```python
from build123d import *

# Parameters (mm, degrees)
SKETCH2_OUTSIDE_W   = 82.784
SKETCH2_OUTSIDE_H   = 82.784
SKETCH2_OUTSIDE_W_2 = 55
SKETCH2_OUTSIDE_H_2 = 76.69931098
CUT_EXTRUDE1_DEPTH  = 17
SKETCH3_W           = 8
SKETCH3_H           = 7.464974998
SKETCH4_R           = 12.75
CUT_EXTRUDE2_DEPTH  = 1


with BuildPart() as part:
    # Sketch1 → Revolve1 (revolve)
    with BuildSketch(Plane.XY, mode=Mode.PRIVATE) as revolve1_sk:
        Polygon((0, 12.5), (60, 12.5), (60, 22.85), (58, 24.85), (55, 24.85), (55, 21.35), (51, 21.35), (51, 24.85), (47.5, 24.85), (47.5, 21.35), (43.5, 21.35), (43.5, 24.85), (38, 24.85), (38, 27), (37.5, 26), (36.75, 27.5), (36, 26), (35.25, 27.5), (34.5, 26), (33.75, 27.5), (33, 26), (32.25, 27.5), (31.5, 26), (30.75, 27.5), (30, 26), (29.25, 27.5), (28.5, 26), (27.75, 27.5), (27, 26), (26.25, 27.5), (25.5, 26), (24.75, 27.5), (24, 26), (23.25, 27.5), (22.5, 26), (21.75, 27.5), (21, 26), (20.25, 27.5), (19.5, 26), (18.75, 27.5), (18, 26), (15, 26), (15, 30), (0, 30), align=None)
    revolve(revolve1_sk.sketch.rotate(Axis((0, 0, 0), (1, 0, 0)), 90), axis=Axis((0, 0, 0), (1, 0, 0)))

    # Sketch2 outside → Cut-Extrude1 (cut)
    with BuildSketch(Plane.ZY):
        Rectangle(SKETCH2_OUTSIDE_W, SKETCH2_OUTSIDE_H)
        Rectangle(SKETCH2_OUTSIDE_W_2, SKETCH2_OUTSIDE_H_2, mode=Mode.SUBTRACT)
    extrude(amount=-CUT_EXTRUDE1_DEPTH, mode=Mode.SUBTRACT)

    # Sketch3 → Cut-Revolve1 (revolve, cut)
    with BuildSketch(Plane(origin=(0, 0, 0), x_dir=(1, 0, 0), z_dir=(0, 1, 0)), mode=Mode.PRIVATE) as cut_revolve1_sk:
        Polygon((4.128668244, 15), (4.128668244, 11.219915318), (0.128668244, 11.219915318), (0.128668244, 12.5), (0.526906778, 15), align=None)
        with Locations((18.128668244, 14.267512501)):
            Rectangle(SKETCH3_W, SKETCH3_H)
        Polygon((32.128668244, 12.5), (32.128668244, 11.219915318), (42.128668244, 11.219915318), (42.128668244, 12.5), (42.128668244, 14.5), (32.128668244, 14.5), align=None)
    revolve(cut_revolve1_sk.sketch.rotate(Axis((0, 0, 0), (1, 0, 0)), 180), axis=Axis((0, 0, 0), (1, 0, 0)), mode=Mode.SUBTRACT)

    # Sketch4 → Cut-Extrude2 (cut)
    with BuildSketch(Plane.ZY):
        Circle(SKETCH4_R)
    extrude(amount=-CUT_EXTRUDE2_DEPTH, mode=Mode.SUBTRACT)


solid = part.part
```
For this review, take the finished solid that the model builds, in its own axes (mm). A direction names the side the tool comes from. Round coordinates to 2 decimals unless told otherwise and drop trailing zeros. Write each loop counter-clockwise with the first axis right and the second up, starting at its lowest first coordinate (ties: lowest second). Pieces come first, ordered by that corner, then holes.
1) Take a section at A-A on x = 10.5. Give the boundary of the cut face in (y, z).
Answer below:
outline: (-11.99, -27.5) - (11.99, -27.5) arc R30 ccw to (11.99, 27.5) - (-11.99, 27.5) arc R30 ccw to start; hole circle Ø25 at (0, 0)
2) Take a section at C-C on x = 48.5. Give the boundary of the cut face in (y, z).
Answer below:
outline: circle Ø49.7 at (0, 0); hole circle Ø25 at (0, 0)
3) For line 1 along Y through (x, z) = (11, 0); line 2 along X through (y, z) = (-16.5, -5); line 3 along Y through (x, z) = (2, 0), list the stretches that pass through material, from the lowest coordinate up.
Answer below:
line 1: y = -30 to -12.5, 12.5 to 30
line 2: x = 0 to 14.13, 22.13 to 60
line 3: y = -30 to -15, 15 to 30
4) Insertion check: pin 1 Ø23 at (y, z) = (0, 0) entering from -X; pin 2 Ø4 at (x, z) = (10, 8.5) entering from -Y; pin 3 Ø1 at (x, z) = (39, -11) entering from +Y. Each pin has a flat end and moves straight along its axis. Give the tip position at first contact, or say it passes through.
Answer below:
pin 1: passes through
pin 2: stops at y = -29.29
pin 3: stops at y = 22.52
5) Machinability: for faces 3 (the face through (7, 0, 27.5)), 4 (the face through (42.129, -7, 11)), 5 (the face through (49.23, 15.12, -19.72)), which of the approach directions +Z, -Z, +X, -X, +Y, -Y give a long, thin tool a straight path to every point of the face, cutting with its end or side? Answer none if there is none.
Answer below:
face 3: +Z, +X, -X, +Y, -Y
face 4: none
face 5: +X
6) Take a section at B-B on x = 16.5. Give the boundary of the cut face in (y, z).
Answer below:
outline: circle Ø52 at (0, 0); hole circle Ø36 at (0, 0)
7) Mouldability with a two-part tool opening along X and no side actions: class faces 1 (the face through (7, -30, 0)), 2 (the face through (14.129, 3.7, 12.3)) as +X half, -X half, draft (parallel to the pull), parting line (faces both ways), or undercut.
Answer below:
face 1: draft
face 2: undercut
